Could you check a few things on this model? Use its own coordinates, in mm. A direction names the side the tool comes from. Round coordinates to 2 decimals unless told otherwise and drop trailing zeros.
```python
from build123d import *

# Parameters (mm, degrees)
F0_W     = 68.5800015926
F0_H     = 74.2950029671
F1_DEPTH = 5


with BuildPart() as f1:
    # F0 (on Front) → F1 (new body)
    with BuildSketch(Plane.XZ):
        with Locations((-0.6015785038, -5.2638160996)):
            Rectangle(F0_W, F0_H)
        with BuildLine():
            add(Edge.make_bspline(
                [(-17.999325617, -7.2772391204), (-18.7571088854, -10.9096900915), (-22.0459496295, -10.9096900915)],
                knots=[0, 0, 0, 1, 1, 1], degree=2))
            add(Edge.make_bspline(
                [(-22.0459496295, -10.9096900915), (-23.0522367228, -10.9096900915), (-23.5124289911, -10.670390112)],
                knots=[0, 0, 0, 1, 1, 1], degree=2))
            Line((-23.5124289911, -10.670390112), (-23.4541379705, -9.262201771))
            add(Edge.make_bspline(
                [(-23.4541379705, -9.262201771), (-22.7945290526, -9.4524145752), (-22.0643573202, -9.4524145752)],
                knots=[0, 0, 0, 1, 1, 1], degree=2))
            add(Edge.make_bspline(
                [(-22.0643573202, -9.4524145752), (-21.1071574022, -9.4524145752), (-20.4782279689, -8.8541646264)],
                knots=[0, 0, 0, 1, 1, 1], degree=2))
            add(Edge.make_bspline(
                [(-20.4782279689, -8.8541646264), (-19.8492985355, -8.2559146776), (-19.609998556, -7.1023660585)],
                knots=[0, 0, 0, 1, 1, 1], degree=2))
            Line((-19.609998556, -7.1023660585), (-16.6678359874, 6.7985083924))
            Line((-16.6678359874, 6.7985083924), (-15.0356874092, 6.7985083924))
            Line((-15.0356874092, 6.7985083924), (-17.999325617, -7.2772391204))
        make_face(mode=Mode.SUBTRACT)
        with BuildLine():
            add(Edge.make_bspline(
                [(-8.9703533131, -7.2434916874), (-9.6606417155, -7.4122288524), (-10.4920557469, -7.4122288524)],
                knots=[0, 0, 0, 1, 1, 1], degree=2))
            add(Edge.make_bspline(
                [(-10.4920557469, -7.4122288524), (-12.2561261087, -7.4122288524), (-13.2639471763, -6.3660584292)],
                knots=[0, 0, 0, 1, 1, 1], degree=2))
            add(Edge.make_bspline(
                [(-13.2639471763, -6.3660584292), (-14.2717682438, -5.3198880059), (-14.2717682438, -3.4699150874)],
                knots=[0, 0, 0, 1, 1, 1], degree=2))
            add(Edge.make_bspline(
                [(-14.2717682438, -3.4699150874), (-14.2717682438, -1.6690293442), (-13.5569362537, -0.0138711525)],
                knots=[0, 0, 0, 1, 1, 1], degree=2))
            add(Edge.make_bspline(
                [(-13.5569362537, -0.0138711525), (-12.8421042637, 1.6412870391), (-11.6624780826, 2.5616715757)],
                knots=[0, 0, 0, 1, 1, 1], degree=2))
            add(Edge.make_bspline(
                [(-11.6624780826, 2.5616715757), (-10.4828519015, 3.4820561123), (-9.0654597152, 3.4820561123)],
                knots=[0, 0, 0, 1, 1, 1], degree=2))
            add(Edge.make_bspline(
                [(-9.0654597152, 3.4820561123), (-7.5989803536, 3.4820561123), (-6.8596047759, 2.8439228336)],
                knots=[0, 0, 0, 1, 1, 1], degree=2))
            add(Edge.make_bspline(
                [(-6.8596047759, 2.8439228336), (-6.1202291981, 2.2057895549), (-6.1202291981, 1.0645127295)],
                knots=[0, 0, 0, 1, 1, 1], degree=2))
            add(Edge.make_bspline(
                [(-6.1202291981, 1.0645127295), (-6.1202291981, -0.6596743024), (-7.7124944464, -1.6429517823)],
                knots=[0, 0, 0, 1, 1, 1], degree=2))
            add(Edge.make_bspline(
                [(-7.7124944464, -1.6429517823), (-9.3047596947, -2.6262292622), (-12.2683979025, -2.6262292622)],
                knots=[0, 0, 0, 1, 1, 1], degree=2))
            Line((-12.2683979025, -2.6262292622), (-12.5843965934, -2.6262292622))
            Line((-12.5843965934, -2.6262292622), (-12.6212119749, -3.393216376))
            add(Edge.make_bspline(
                [(-12.6212119749, -3.393216376), (-12.6212119749, -4.6480072942), (-12.0321658715, -5.353635439)],
                knots=[0, 0, 0, 1, 1, 1], degree=2))
            add(Edge.make_bspline(
                [(-12.0321658715, -5.353635439), (-11.443119768, -6.0592635837), (-10.2067365406, -6.0592635837)],
                knots=[0, 0, 0, 1, 1, 1], degree=2))
            add(Edge.make_bspline(
                [(-10.2067365406, -6.0592635837), (-9.6023506949, -6.0592635837), (-8.9642174162, -5.8859244959)],
                knots=[0, 0, 0, 1, 1, 1], degree=2))
            add(Edge.make_bspline(
                [(-8.9642174162, -5.8859244959), (-8.3260841375, -5.7125854082), (-7.3780880648, -5.2523931399)],
                knots=[0, 0, 0, 1, 1, 1], degree=2))
            Line((-7.3780880648, -5.2523931399), (-7.3780880648, -6.654445584))
            add(Edge.make_bspline(
                [(-7.3780880648, -6.654445584), (-8.2800649107, -7.0747545224), (-8.9703533131, -7.2434916874)],
                knots=[0, 0, 0, 1, 1, 1], degree=2))
        make_face(mode=Mode.SUBTRACT)
        with BuildLine():
            add(Edge.make_bspline(
                [(-2.029119933, 2.5125844004), (-0.8310860612, 3.4820561123), (0.5985779189, 3.4820561123)],
                knots=[0, 0, 0, 1, 1, 1], degree=2))
            add(Edge.make_bspline(
                [(0.5985779189, 3.4820561123), (1.4790791256, 3.4820561123), (2.169367528, 3.0065241017)],
                knots=[0, 0, 0, 1, 1, 1], degree=2))
            add(Edge.make_bspline(
                [(2.169367528, 3.0065241017), (2.8596559305, 2.5309920911), (3.2431494874, 1.6412870391)],
                knots=[0, 0, 0, 1, 1, 1], degree=2))
            Line((3.2431494874, 1.6412870391), (3.3505276833, 1.6412870391))
            Line((3.3505276833, 1.6412870391), (3.9917289105, 3.2887753596))
            Line((3.9917289105, 3.2887753596), (5.2097044472, 3.2887753596))
            Line((5.2097044472, 3.2887753596), (2.9762379718, -7.2189480998))
            Line((2.9762379718, -7.2189480998), (1.6999714144, -7.2189480998))
            Line((1.6999714144, -7.2189480998), (1.9515431877, -5.2155777585))
            Line((1.9515431877, -5.2155777585), (1.8748444763, -5.2155777585))
            add(Edge.make_bspline(
                [(1.8748444763, -5.2155777585), (0.1567933414, -7.4122288524), (-1.7422667524, -7.4122288524)],
                knots=[0, 0, 0, 1, 1, 1], degree=2))
            add(Edge.make_bspline(
                [(-1.7422667524, -7.4122288524), (-3.073756382, -7.4122288524), (-3.8315396505, -6.4626988055)],
                knots=[0, 0, 0, 1, 1, 1], degree=2))
            add(Edge.make_bspline(
                [(-3.8315396505, -6.4626988055), (-4.5893229189, -5.5131687586), (-4.5893229189, -3.8626124897)],
                knots=[0, 0, 0, 1, 1, 1], degree=2))
            add(Edge.make_bspline(
                [(-4.5893229189, -3.8626124897), (-4.5893229189, -1.8684459938), (-3.9082383619, -0.1626666526)],
                knots=[0, 0, 0, 1, 1, 1], degree=2))
            add(Edge.make_bspline(
                [(-3.9082383619, -0.1626666526), (-3.2271538048, 1.5431126885), (-2.029119933, 2.5125844004)],
                knots=[0, 0, 0, 1, 1, 1], degree=2))
        make_face(mode=Mode.SUBTRACT)
        with BuildLine():
            Line((14.1834536789, -7.2189480998), (12.5543730492, -7.2189480998))
            Line((12.5543730492, -7.2189480998), (13.974833184, -0.582975591))
            add(Edge.make_bspline(
                [(13.974833184, -0.582975591), (14.1650459882, 0.414107657), (14.1650459882, 0.7976012139)],
                knots=[0, 0, 0, 1, 1, 1], degree=2))
            add(Edge.make_bspline(
                [(14.1650459882, 0.7976012139), (14.1650459882, 1.3989191111), (13.8245037097, 1.7640049773)],
                knots=[0, 0, 0, 1, 1, 1], degree=2))
            add(Edge.make_bspline(
                [(13.8245037097, 1.7640049773), (13.4839614311, 2.1290908435), (12.7384499565, 2.1290908435)],
                knots=[0, 0, 0, 1, 1, 1], degree=2))
            add(Edge.make_bspline(
                [(12.7384499565, 2.1290908435), (11.8824923375, 2.1290908435), (11.0725539453, 1.5538505081)],
                knots=[0, 0, 0, 1, 1, 1], degree=2))
            add(Edge.make_bspline(
                [(11.0725539453, 1.5538505081), (10.2626155531, 0.9786101728), (9.6444239393, -0.0859679412)],
                knots=[0, 0, 0, 1, 1, 1], degree=2))
            add(Edge.make_bspline(
                [(9.6444239393, -0.0859679412), (9.0262323256, -1.1505460552), (8.7102336347, -2.6661125921)],
                knots=[0, 0, 0, 1, 1, 1], degree=2))
            Line((8.7102336347, -2.6661125921), (7.7407619228, -7.2189480998))
            Line((7.7407619228, -7.2189480998), (6.1300889838, -7.2189480998))
            Line((6.1300889838, -7.2189480998), (8.3758272531, 3.2887753596))
            Line((8.3758272531, 3.2887753596), (9.7073168827, 3.2887753596))
            Line((9.7073168827, 3.2887753596), (9.4956284393, 1.3436960389))
            Line((9.4956284393, 1.3436960389), (9.5938027898, 1.3436960389))
            add(Edge.make_bspline(
                [(9.5938027898, 1.3436960389), (10.5141873264, 2.5125844004), (11.3716789197, 2.9973202563)],
                knots=[0, 0, 0, 1, 1, 1], degree=2))
            add(Edge.make_bspline(
                [(11.3716789197, 2.9973202563), (12.2291705129, 3.4820561123), (13.1495550495, 3.4820561123)],
                knots=[0, 0, 0, 1, 1, 1], degree=2))
            add(Edge.make_bspline(
                [(13.1495550495, 3.4820561123), (14.3675305862, 3.4820561123), (15.0716247567, 2.8147773232)],
                knots=[0, 0, 0, 1, 1, 1], degree=2))
            add(Edge.make_bspline(
                [(15.0716247567, 2.8147773232), (15.7757189272, 2.1474985342), (15.7757189272, 0.9509986367)],
                knots=[0, 0, 0, 1, 1, 1], degree=2))
            add(Edge.make_bspline(
                [(15.7757189272, 0.9509986367), (15.7757189272, 0.1932153682), (15.5548266384, -0.7762563437)],
                knots=[0, 0, 0, 1, 1, 1], degree=2))
            Line((15.5548266384, -0.7762563437), (14.1834536789, -7.2189480998))
        make_face(mode=Mode.SUBTRACT)
    extrude(amount=F1_DEPTH)


solid = f1.part
```
Q1. We'd pull the mould along X, two halves only. Please class faces 3 (the flat face through (-1, -2, 31.884)), 4 (the flat face through (-34.892, -2, -6)), 5 (the flat face through (9.6, -2.5, 2.3)): released by +X, released by -X, zero draft, split by the parting line, or undercut.
Q2. I need wall thicknesses on L1, parallel to X at y = -1.6, z = -1.5 (3 decimals); L2, parallel to X at y = -1.15, z = -1; L3, parallel to Z at x = -6.5, y = -2.95. Which ranges of each line are inside material? Lowest first, please.
Q3. Imagine slicing it at A-A, the plane y = -0.95. State how many separate pieces and enclosed holes the cut face has, then the cut area to 3 significant figures.
Q4. For faces 1 (the flat face through (-1, -2, -42.411)), 2 (the flat face through (4.11, -2.46, -1.89)), which set-ups out of +Z, -Z, +X, -X, +Y, -Y let a thin tool reach every point of the face, with its end or its side?
Filled in:
1. face 3: zero draft
1. face 4: released by -X
1. face 5: undercut
2. L1: x = -34.892 to -18.424, -16.783 to -14.048, -7.495 to -4.327, 4.192 to 7.352, 9.02 to 13.779, 15.401 to 33.688
2. L2: x = -34.89 to -18.32, -16.68 to -13.92, -6.91 to -4.2, 4.3 to 7.46, 9.2 to 13.89, 15.51 to 33.69
2. L3: z = -42.41 to -0.44, 2.44 to 31.88
3. separate pieces: 1
3. enclosed holes: 4
3. area: 4,890 mm2
4. face 1: -Z, +X, -X, +Y, -Y
4. face 2: +Y, -Y
